Design review of the part shown in the three views and the two pictorial views. Dimensions are in mm from the part's minimum x, y and z. Give positions to 0.01 mm unless a question says otherwise; leave off trailing zeros. Loops run counter-clockwise (first coordinate to the right, second up) from the corner with the lowest first, then second, coordinate; pieces in that order, holes last. Notation, with made-up numbers: (21, 47.5) -> (36, 47.5) arc R33 ccw to (36, 86.5) -> close; hole circle Ø1 at (56.25, 61). An arc over 180 degrees is marked (long way). Answer as CSV lines item,"result". Start each with the question number.
Item 1: Add section C-C on z = 1. State the section outline as (x, y) points (3 decimals).
Item 2: Clearance check with flat-ended pins moving along their axes: P1, Ø1.9, axis at y = 90.5, z = 4, coming from the +X side; P2, Ø2, axis at x = 67.5, z = 3.5, coming from the +Y side; P3, Ø1, axis at y = 106.5, z = 0.5, coming from the +X side. State where each tip first meets the part, or that it passes through.
Item 3: For L1, parallel to X at y = 94, z = 2.5 (3 decimals); L2, parallel to Y at x = 61, z = 0.75 (3 decimals); L3, parallel to Y at x = 88.5, z = 2 (3 decimals), list the stretches that pass through material, from the lowest coordinate up. Write a range as from..to.
Item 4: Add section D-D on x = 16. State the section outline as (y, z) points.
Item 5: Add section A-A on y = 76.2. State the section outline as (x, z) points (3 decimals), plus the area to 3 significant figures.
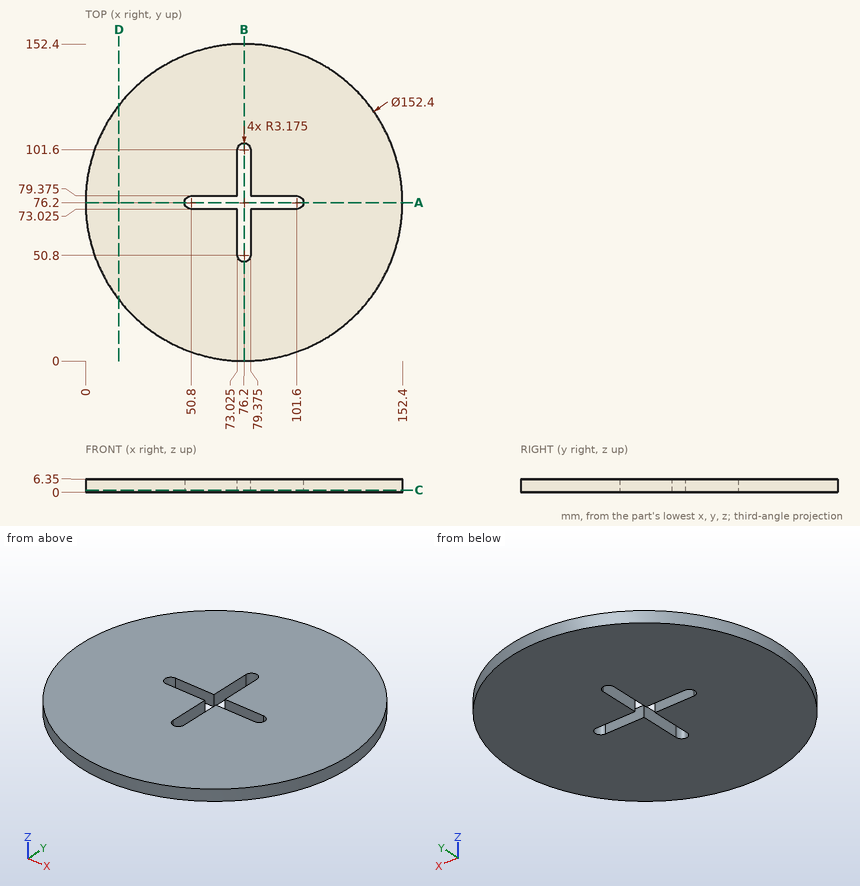
Computed values:
1,outline,"circle Ø152.4 at (76.2, 76.2); hole (50.8, 73.025) -> (73.025, 73.025) -> (73.025, 50.8) arc R3.175 ccw to (79.375, 50.8) -> (79.375, 73.025) -> (101.6, 73.025) arc R3.175 ccw to (101.6, 79.375) -> (79.375, 79.375) -> (79.375, 101.6) arc R3.175 ccw to (73.025, 101.6) -> (73.025, 79.375) -> (50.8, 79.375) arc R3.175 ccw to start"
2,P1,"x = 151.22"
2,P2,"y = 152.01"
2,P3,"x = 146.33"
3,L1,"2.108..73.025, 79.375..150.292"
3,L2,"1.531..73.025, 79.375..150.869"
3,L3,"0.999..73.025, 79.375..151.401"
4,outline,"(29.48, 0) -> (122.92, 0) -> (122.92, 6.35) -> (29.48, 6.35) -> close"
5,outline,"(0, 0) -> (47.625, 0) -> (47.625, 6.35) -> (0, 6.35) -> close; (104.775, 0) -> (152.4, 0) -> (152.4, 6.35) -> (104.775, 6.35) -> close"
5,area,"605 mm²"
